Work out the finished part from the listing and answer in its coordinate system (mm). Round coordinates to 2 decimals unless told otherwise and drop trailing zeros. Write each loop counter-clockwise with the first axis right and the second up, starting at its lowest first coordinate (ties: lowest second). Pieces come first, ordered by that corner, then holes. Notation, with made-up numbers: (-38.5, 20.5) -> (1.5, 20.5) arc R4 cw to (1.5, 26.5) -> close; hole circle Ø9 at (63, 21.5). An arc over 180 degrees is marked (long way). One line per item, written item: value.
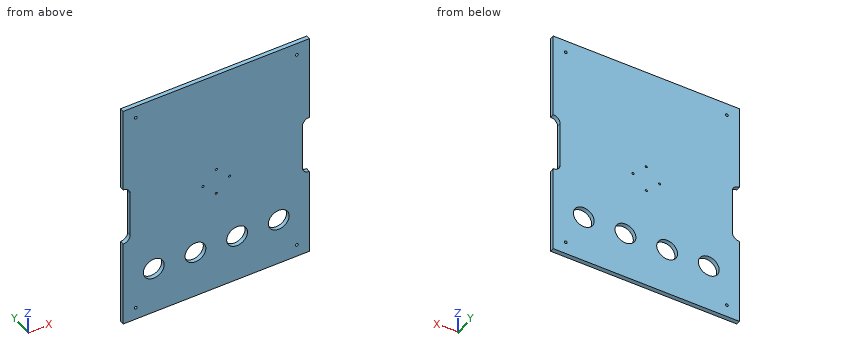
```python
from build123d import *

# Parameters (mm, degrees)
RESSALTO_EXTRUS_O1_DEPTH     = 6
FURO_ROSCADO_DE_M41_D        = 3
ESBO_O6_R                    = 15
CORTE_EXTRUS_O1_DEPTH        = 216.761442339
FURO_DE_DI_METRO_4_2_4_2_1_D = 4.2


with BuildPart() as part:
    # Esboço1 → Ressalto-extrusão1 (new body)
    with BuildSketch(Plane(origin=(0, 0, 0), x_dir=(1, 0, 0), z_dir=(0, 1, 0))):
        with BuildLine():
            Line((-134, -169), (134, -169))
            Line((134, -169), (134, -44))
            ThreePointArc((134, -44), (126.928932188, -41.071067812), (124, -34))
            Line((124, -34), (124, 32))
            ThreePointArc((124, 32), (126.928932188, 39.071067812), (134, 42))
            Line((134, 42), (134, 169))
            Line((134, 169), (-134, 169))
            Line((-134, 169), (-134, 42))
            ThreePointArc((-134, 42), (-126.928932188, 39.071067812), (-124, 32))
            Line((-124, 32), (-124, -34))
            ThreePointArc((-124, -34), (-126.928932188, -41.071067812), (-134, -44))
            Line((-134, -44), (-134, -169))
        make_face()
    extrude(amount=RESSALTO_EXTRUS_O1_DEPTH)

    # Furo roscado de M41 (through all)
    with Locations(Plane(origin=(0, 0, 0), x_dir=(-1, 0, 0), z_dir=(0, -1, 0))):
        with Locations((19, 0), (0, 19), (-19, 0), (0, -19)):
            Hole(FURO_ROSCADO_DE_M41_D / 2)

    # Esboço6 → Corte-extrusão1 (cut, through all)
    with BuildSketch(Plane(origin=(0, 6, 0), x_dir=(1, 0, 0), z_dir=(0, 1, 0))):
        with Locations(Location((-90, 100, 0), (0, 0, 270))):
            Circle(ESBO_O6_R)
        with Locations(Location((-30, 100, 0), (0, 0, 270))):
            Circle(ESBO_O6_R)
        with Locations(Location((30, 100, 0), (0, 0, 270))):
            Circle(ESBO_O6_R)
        with Locations(Location((90, 100, 0), (0, 0, 270))):
            Circle(ESBO_O6_R)
    extrude(amount=-CORTE_EXTRUS_O1_DEPTH, mode=Mode.SUBTRACT)

    # Furo de diâmetro Ø4.2 (4.2)1 (through all)
    with Locations(Plane(origin=(0, 0, 0), x_dir=(-1, 0, 0), z_dir=(0, -1, 0))):
        with Locations((-116, 151), (-116, -151), (116, 151), (116, -151)):
            Hole(FURO_DE_DI_METRO_4_2_4_2_1_D / 2)


solid = part.part
```
(1) Find section A-A on z = -100. Give the vertices of the cut face in (x, y).
Reported:
outline: (-134, 0) -> (-105, 0) -> (-105, 6) -> (-134, 6) -> close; (-75, 0) -> (-45, 0) -> (-45, 6) -> (-75, 6) -> close; (-15, 0) -> (15, 0) -> (15, 6) -> (-15, 6) -> close; (45, 0) -> (75, 0) -> (75, 6) -> (45, 6) -> close; (105, 0) -> (134, 0) -> (134, 6) -> (105, 6) -> close
(2) Find section B-B on y = 1.9. Give the number of separate pieces and of enclosed holes in the cut face, plus the area to 3 significant figures.
Reported:
separate pieces: 1
enclosed holes: 12
area: 86,000 mm2
(3) Find section D-D on z = 7.5. Give the vertices of the cut face in (x, y).
Reported:
outline: (-124, 0) -> (124, 0) -> (124, 6) -> (-124, 6) -> close
(4) Flat-ended cylindrical pins translate along their axes: pin 1 Ø3.5 at (x, z) = (116, 151) entering from +Y; pin 2 Ø1.8 at (y, z) = (2.5, -5) entering from +X. Find the tip coordinate at first contact, or state that the pin passes through.
Reported:
pin 1: passes through
pin 2: stops at x = 124
(5) Find section C-C on x = -30. Give the vertices of the cut face in (y, z).
Reported:
outline: (0, -169) -> (6, -169) -> (6, -115) -> (0, -115) -> close; (0, -85) -> (6, -85) -> (6, 169) -> (0, 169) -> close
(6) Consider probe 1 along X at (y, z) = (3, 151); probe 2 along X at (y, z) = (1.6, -100); probe 3 along Z at (x, y) = (29.5, 0.7). Determine where each line is inside the solid, lowest interval first.
Reported:
probe 1: x = -134 to -118.1, -113.9 to 113.9, 118.1 to 134
probe 2: x = -134 to -105, -75 to -45, -15 to 15, 45 to 75, 105 to 134
probe 3: z = -169 to -114.99, -85.01 to 169
